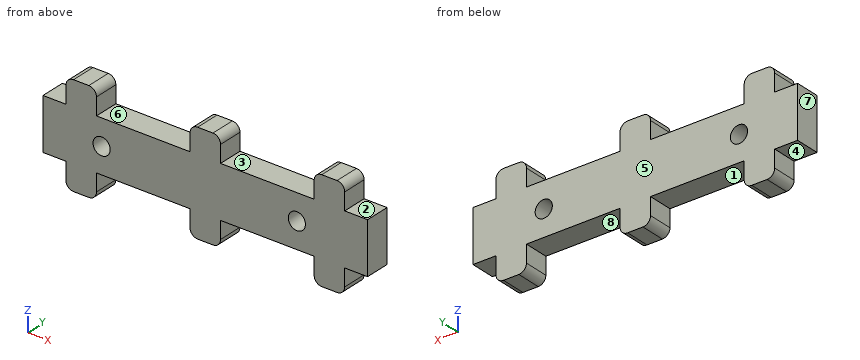
Autodesk Inventor part; units mm, degrees
ref_plane "YZ Plane" through (0, 0, 0) normal (1, 0, 0) x (0, 1, 0)
ref_plane "XZ Plane" through (0, 0, 0) normal (0, 1, 0) x (-1, 0, 0)
ref_plane "XY Plane" through (0, 0, 0) normal (0, 0, 1) x (1, 0, 0)
sketch "Sketch1" plane through (0, 0, 0) normal (0, 1, 0) x (-1, 0, 0)
  line L0 (0, 0) -> (-85, 0)
  line L1 (-85, 0) -> (-85, -13.5)
  line L2 (-85, -13.5) -> (0, -13.5)
  line L3 (0, -13.5) -> (0, 0)
  dimension "d0" = 85
  dimension "d1" = 13.5
extrude "Extrusion1" add sketch "Sketch1" along normal blind 6.5
sketch "Sketch2" plane through (0, 6.5, 0) normal (0, 1, 0) x (1, 0, 0)
  line L0 (0, 0) -> (85, 0)
  line L1 (85, 0) -> (85, 13.5)
  line L2 (85, 13.5) -> (0, 13.5)
  line L3 (0, 13.5) -> (0, 0)
  line L4 (6, 13.5) -> (14, 13.5)
  line L5 (14, 13.5) -> (14, 18)
  line L6 (12, 20) -> (8, 20)
  line L7 (6, 18) -> (6, 13.5)
  line L8 (38.5, 13.5) -> (46.5, 13.5)
  line L9 (46.5, 13.5) -> (46.5, 18)
  line L10 (44.5, 20) -> (40.5, 20)
  line L11 (38.5, 18) -> (38.5, 13.5)
  line L12 (71, 13.5) -> (79, 13.5)
  line L13 (79, 13.5) -> (79, 18)
  line L14 (77, 20) -> (73, 20)
  line L15 (71, 18) -> (71, 13.5)
  line L16 (6, 0) -> (14, 0)
  line L17 (14, 0) -> (14, -4.5)
  line L18 (12, -6.5) -> (8, -6.5)
  line L19 (6, -4.5) -> (6, 0)
  line L20 (38.5, 0) -> (46.5, 0)
  line L21 (46.5, 0) -> (46.5, -4.5)
  line L22 (44.5, -6.5) -> (40.5, -6.5)
  line L23 (38.5, -4.5) -> (38.5, 0)
  line L24 (71, 0) -> (79, 0)
  line L25 (79, 0) -> (79, -4.5)
  line L26 (77, -6.5) -> (73, -6.5)
  line L27 (71, -4.5) -> (71, 0)
  arc A0 (8, 20) -> (6, 18) centre (8, 18) ccw
  arc A1 (14, 18) -> (12, 20) centre (12, 18) ccw
  arc A2 (40.5, 20) -> (38.5, 18) centre (40.5, 18) ccw
  arc A3 (46.5, 18) -> (44.5, 20) centre (44.5, 18) ccw
  arc A4 (73, 20) -> (71, 18) centre (73, 18) ccw
  arc A5 (79, 18) -> (77, 20) centre (77, 18) ccw
  arc A6 (6, -4.5) -> (8, -6.5) centre (8, -4.5) ccw
  arc A7 (12, -6.5) -> (14, -4.5) centre (12, -4.5) ccw
  arc A8 (38.5, -4.5) -> (40.5, -6.5) centre (40.5, -4.5) ccw
  arc A9 (44.5, -6.5) -> (46.5, -4.5) centre (44.5, -4.5) ccw
  arc A10 (71, -4.5) -> (73, -6.5) centre (73, -4.5) ccw
  arc A11 (77, -6.5) -> (79, -4.5) centre (77, -4.5) ccw
  line L28 (14, 15.75) -> (38.5, 15.75) construction
  line L29 (46.5, 15.75) -> (71, 15.75) construction
  dimension "d4" = 2
  dimension "d5" = 8
  dimension "d6" = 8
  dimension "d7" = 8
  dimension "d8" = 6.5
  dimension "d9" = 6.5
  dimension "d10" = 6
  dimension "d11" = 6
extrude "Extrusion2" add sketch "Sketch2" against normal blind 6.5 contours L0 L17 A7 L18 A6 L19 | L7 A0 L6 A1 L5 L2 | L0 L21 A9 L22 A8 L23 | L11 A2 L10 A3 L9 L2 | L0 L25 A11 L26 A10 L27 | L15 A4 L14 A5 L13 L2
sketch "Sketch4" plane through (0, 6.5, 0) normal (0, 1, 0) x (1, 0, 0)
  line L0 (85, 0) -> (85, 13.5)
  circle A0 centre (66.4711, 6.75) radius 2.25
  line L1 (46.5, 0) -> (71, 0)
  line L2 (85, 0) -> (0, -27.6346) construction
  line L3 (71, 13.5) -> (46.5, 13.5)
  line L4 (70.2271, -4.8028) -> (64.2766, 13.5) construction
  point P0 (85, 6.75)
  point P1 (0, 0)
  dimension "d14" = 4.5
  dimension "d18" = 18.01
  dimension "d19" = 15.534
extrude "Extrusion3" cut sketch "Sketch4" against normal through all
sketch "Sketch5" plane through (0, 6.5, 0) normal (0, 1, 0) x (1, 0, 0)
  circle A0 centre (66.4711, 6.75) radius 2.25
  line L0 (85, 0) -> (85, 13.5)
  line L1 (0, 13.5) -> (0, 0)
  circle A1 centre (15.354, 6.75) radius 2.25
  point P0 (0, 6.75)
  dimension "d22" = 69.646
extrude "Extrusion4" cut sketch "Sketch5" against normal through all contours A1
equation "\"d6\" = d5"
equation "\"d7\" = d6"
equation "\"d9\" = d8"
equation "\"d11\" = d10"
properties part number "z_pulley_holder" material "Plywood, Finish"
Work out the finished part from the listing and answer in its coordinate system (mm). Face numbers are marked on the shaded views. A direction names the side the tool comes from. Round coordinates to 2 decimals unless told otherwise and drop trailing zeros. Loops run counter-clockwise (first coordinate to the right, second up) from the corner with the lowest first, then second, coordinate; pieces in that order, holes last. Notation, with made-up numbers: (-31, 9) - (-2, 9) arc R16 cw to (-2, 29) - close; hole circle Ø2 at (15.25, 34). An arc over 180 degrees is marked (long way). One line per item, written item: value.
Q1. Find section A-A on z = -17. Give the vertices of the cut face in (x, y).
Check values:
outline: (6, 0) - (14, 0) - (14, 6.5) - (6, 6.5) - close; (38.5, 0) - (46.5, 0) - (46.5, 6.5) - (38.5, 6.5) - close; (71, 0) - (79, 0) - (79, 6.5) - (71, 6.5) - close
Q2. Find section C-C on z = -6.75. Give the vertices of the cut face in (x, y), and give its area (3 significant figures).
Check values:
outline: (0, 0) - (13.1, 0) - (13.1, 6.5) - (0, 6.5) - close; (17.6, 0) - (64.22, 0) - (64.22, 6.5) - (17.6, 6.5) - close; (68.72, 0) - (85, 0) - (85, 6.5) - (68.72, 6.5) - close
area: 494 mm2
Q3. Each of these flat-tipped pins is pushed along its axis until it touches: pin 1 Ø2 at (x, y) = (30, 4) entering from +Z; pin 2 Ø3.5 at (y, z) = (2, -16) entering from +X; pin 3 Ø2 at (x, y) = (62.5, 1.5) entering from -Z. Where does it stop, or does it pass through?
Check values:
pin 1: z = 0
pin 2: x = 79
pin 3: z = -13.5
Q4. For the marked faces 1, 2, 3 and 4, determine the directions among +Z, -Z, +X, -X, +Y, -Y from which every point of the face is accessible in a straight line to the end or side of a thin tool.
Check values:
face 1: -Z, +Y, -Y
face 2: +Z, +X, +Y, -Y
face 3: +Z, +Y, -Y
face 4: -Z, -X, +Y, -Y
Q5. The mould has two halves that part along X. Classify the marked faces 5, 6, 7 and 8: +X half, -X half, draft (parallel to the pull), parting line (faces both ways), or undercut.
Check values:
face 5: draft
face 6: undercut
face 7: -X half
face 8: undercut
Q6. Find section B-B on x = 68. Give the vertices of the cut face in (y, z).
Check values:
outline: (0, -13.5) - (6.5, -13.5) - (6.5, -8.4) - (0, -8.4) - close; (0, -5.1) - (6.5, -5.1) - (6.5, 0) - (0, 0) - close
Q7. Straight lines are drawn through the part: probe 1 along X at (y, z) = (6.25, -18); probe 2 along X at (y, z) = (1.75, -6.75); probe 3 along Z at (x, y) = (61, 2). For each, find the intervals that lie inside material, in ascending order.
Check values:
probe 1: 6 to 14, 38.5 to 46.5, 71 to 79
probe 2: 0 to 13.1, 17.6 to 64.22, 68.72 to 85
probe 3: -13.5 to 0
Q8. Find section D-D on y = 1. State how many separate pieces and enclosed holes the cut face has, and give its area (3 significant figures).
Check values:
separate pieces: 1
enclosed holes: 2
area: 1,420 mm2
